```python
from build123d import *

# Parameters (mm, degrees)
F1_DEPTH = 304.8
F4_DEPTH = 12.7
F5_W     = 127
F5_H     = 165.1
F6_DEPTH = 12.7
F7_R     = 19.05
F7_R_2   = 12.7
F8_DEPTH = 76.2


with BuildPart() as f1:
    # F0 (on Top) → F1 (new body)
    with BuildSketch(Plane.XY):
        Polygon((123.7545942165, 609.6), (123.7545942165, -609.6), (69.8730574901, -663.4815367264), (75.5663116695, -666.7685385595), (130.1045942165, -612.2302560125), (130.1045942165, 612.2302561211), (75.4418789804, 666.8929713571), (69.8730574901, 663.4815367264), align=None)
    extrude(amount=F1_DEPTH)

    # F3 (on offset) → F4 (join)
    with BuildSketch(Plane.XY.offset(76.2)):
        with BuildLine():
            Line((130.1045942165, 101.6), (130.1045942165, -101.6))
            Line((130.1045942165, -101.6), (161.8545942165, -101.6))
            ThreePointArc((161.8545942165, -101.6), (263.4545942165, 0), (161.8545942165, 101.6))
            Line((161.8545942165, 101.6), (130.1045942165, 101.6))
        make_face()
    extrude(amount=F4_DEPTH)

    # F5 (on face) → F6 (join)
    with BuildSketch(Plane(origin=(0, 0, 76.2), x_dir=(1, 0, 0), z_dir=(0, 0, -1))):
        with Locations((244.4045942165, 0)):
            Rectangle(F5_W, F5_H)
    extrude(amount=F6_DEPTH)

    # F7 (on Front) → F8 (join, symmetric)
    with BuildSketch(Plane.XZ):
        with Locations((288.8545942165, 94.615)):
            Circle(F7_R)
        with Locations((288.8545942165, 94.615)):
            Circle(F7_R_2, mode=Mode.SUBTRACT)
    extrude(amount=F8_DEPTH, both=True)


solid = f1.part
```
Work out the finished part from the listing and answer in its coordinate system (mm). A direction names the side the tool comes from. Coordinates: 2 decimals unless noted, no trailing zeros. Order: outer loops, then holes, each group sorted by start corner. A loop starts at its lowest first (then second) coordinate and runs counter-clockwise, first axis right, second up. Notation, with made-up numbers: (-7, 34.5) - (40, 34.5) arc R23 ccw to (40, 59.5) - close; hole circle Ø4 at (56.5, 29). An arc over 180 degrees is marked (long way). Answer as a JSON object with one key per item and string values.
1. Each of these flat-tipped pins is pushed along its axis until it touches: P1, Ø6.5, axis at x = 145.5, z = 82, coming from the -Y side; P2, Ø4, axis at x = 267.5, z = 68.5, coming from the +Y side; P3, Ø3, axis at x = 189.5, z = 72.5, coming from the -Y side. Where does it stop, or does it pass through?
Output values:
{"P1": "stops at y = -101.6", "P2": "stops at y = 82.55", "P3": "stops at y = -82.55"}
2. Find section B-B on x = 100. Determine the outline of the cut face in (y, z).
Output values:
{"outline": "(-642.33, 0) - (-633.35, 0) - (-633.35, 304.8) - (-642.33, 304.8) - close; (633.35, 0) - (642.33, 0) - (642.33, 304.8) - (633.35, 304.8) - close"}
3. A tool of negligible diameter and unlimited length cuts with its end or side. For faces 5 (the face through (263.43, -2.23, 82.46)), 6 (the face through (181, 1, 88.9)), 7 (the face through (244, -1, 63.5)), from which of +Z, -Z, +X, -X, +Y, -Y can it reach the whole face along a straight path? Write none if from no direction.
Output values:
{"face 5": "+Z", "face 6": "+Z, +Y, -Y", "face 7": "-Z, +X, +Y, -Y"}
4. The mould has two halves that part along Y. Classify faces 1 (the face through (276, -76.2, 95)), 2 (the face through (155, 1, 76.2)), 3 (the face through (96.437, 636.918, 150.266)), 4 (the face through (97.191, -636.164, 150.266)): +Y half, -Y half, draft (parallel to the pull), parting line (faces both ways), or undercut.
Output values:
{"face 1": "-Y half", "face 2": "draft", "face 3": "undercut", "face 4": "undercut"}
5. Consider line 1 (Z direction, x = 282.5, y = 15.5); line 2 (X direction, y = 223, z = 48.5); line 3 (Y direction, x = 110, z = 221). Determine where each line is inside the solid, lowest interval first.
Output values:
{"line 1": "z = 63.5 to 76.2, 76.66 to 83.62, 105.61 to 112.57", "line 2": "x = 123.75 to 130.1", "line 3": "y = -632.33 to -623.35, 623.35 to 632.33"}
6. Find section A-A on z = 256. Determine the outline of the cut face in (x, y).
Output values:
{"outline": "(69.87, -663.48) - (75.57, -666.77) - (130.1, -612.23) - (130.1, 612.23) - (75.44, 666.89) - (69.87, 663.48) - (123.75, 609.6) - (123.75, -609.6) - close"}
7. Find section C-C on y = 0. Determine the outline of the cut face in (x, z) (3 decimals).
Output values:
{"outline": "(123.755, 0) - (130.105, 0) - (130.105, 76.2) - (180.905, 76.2) - (180.905, 63.5) - (307.905, 63.5) - (307.905, 76.2) - (293.732, 76.2) arc R19.05 ccw (long way) to (283.977, 76.2) - (263.455, 76.2) - (263.455, 88.9) - (130.105, 88.9) - (130.105, 304.8) - (123.755, 304.8) - close; hole circle Ø25.4 at (288.855, 94.615)"}
8. Find section D-D on y = 235.5. Determine the outline of the cut face in (x, z), plus the area to 3 significant figures.
Output values:
{"outline": "(123.75, 0) - (130.1, 0) - (130.1, 304.8) - (123.75, 304.8) - close", "area": "1,940 mm²"}
